Input: part model. Units: mm. Frame: model coordinates. Coordinates: 2 decimals unless noted, no trailing zeros. Loops run counter-clockwise (first coordinate to the right, second up) from the corner with the lowest first, then second, coordinate; pieces in that order, holes last.
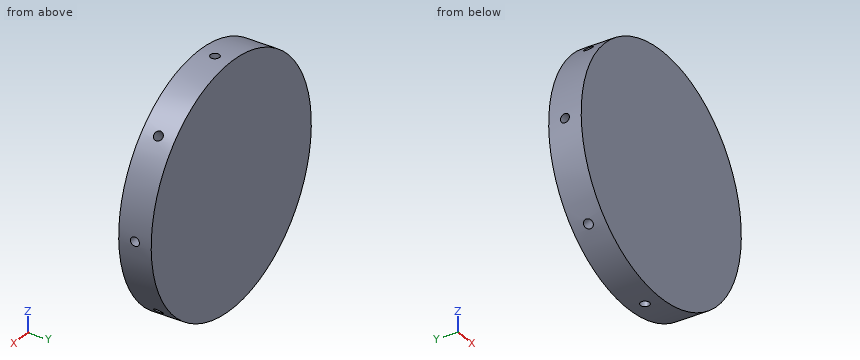
```python
from build123d import *

# Parameters (mm, degrees)
SKETCH1_R           = 46.99
BOSS_EXTRUDE1_DEPTH = 12.7
SKETCH2_R           = 1.7526
CUT_EXTRUDE1_DEPTH  = 19.05
CIRPATTERN1_COUNT   = 8


with BuildPart() as part:
    # Sketch1 → Boss-Extrude1 (new body)
    with BuildSketch(Plane(origin=(0, 0, 0), x_dir=(1, 0, 0), z_dir=(0, 1, 0))):
        with Locations(Location((0, 0, 0), (0, 0, 270))):
            Circle(SKETCH1_R)
    extrude(amount=BOSS_EXTRUDE1_DEPTH)

    # Sketch2 → Cut-Extrude1 (cut)
    with BuildSketch(Plane.XY.offset(46.99)):
        with Locations((0, 6.35)):
            Circle(SKETCH2_R)
    cut_extrude1 = extrude(amount=-CUT_EXTRUDE1_DEPTH, mode=Mode.SUBTRACT)

    # CirPattern1: Cut-Extrude1 ×8 about axis
    cirpattern1_axis = Axis((0, 0, 0), (0, 1, 0))
    for i in range(1, CIRPATTERN1_COUNT):
        add(cut_extrude1.rotate(cirpattern1_axis, i * 360 / CIRPATTERN1_COUNT), mode=Mode.SUBTRACT)


solid = part.part
```
Item 1: Section query A-A (x = 0). Output: boundary loops of the cut face in (y, z).
Result:
outline: (0, -46.99) - (4.6, -46.99) - (4.6, -27.94) - (8.1, -27.94) - (8.1, -46.99) - (12.7, -46.99) - (12.7, 46.99) - (8.1, 46.99) - (8.1, 27.94) - (4.6, 27.94) - (4.6, 46.99) - (0, 46.99) - close
Item 2: Section query B-B (z = 0). Output: boundary loops of the cut face in (x, y).
Result:
outline: (-46.99, 0) - (46.99, 0) - (46.99, 4.6) - (27.94, 4.6) - (27.94, 8.1) - (46.99, 8.1) - (46.99, 12.7) - (-46.99, 12.7) - (-46.99, 8.1) - (-27.94, 8.1) - (-27.94, 4.6) - (-46.99, 4.6) - close
Item 3: Line query: L1, parallel to Y at x = 35, z = 0; L2, parallel to Z at x = -25.5, y = 6.25; L3, parallel to X at y = 6, z = 21.5. Output: solid intervals per line, ascending.
Result:
L1: y = 0 to 4.6, 8.1 to 12.7
L2: z = -39.47 to -27.97, -23.03 to 23.03, 27.97 to 39.47
L3: x = -41.78 to -23.93, -19.07 to 19.07, 23.93 to 41.78
Item 4: Contact query for flat-ended pins moving along their axis: P1, Ø1.8, axis at y = 6.5, z = 0, coming from the +X side; P2, Ø6, axis at y = 5.5, z = -12.5, coming from the -X side; P3, Ø1.8, axis at x = 0, y = 6.5, coming from the +Z side. Output: stop coordinate, or through.
Result:
P1: stops at x = 27.94
P2: stops at x = -46.02
P3: stops at z = 27.94
Item 5: Section query D-D (x = -39). Output: boundary loops of the cut face in (y, z), then the cut area to 3 significant figures.
Result:
outline: (0, -26.21) - (12.7, -26.21) - (12.7, 26.21) - (0, 26.21) - close; hole circle Ø3.51 at (6.35, 0)
area: 656 mm2
